from build123d import *

# Parameters (mm, degrees)
BOSS_EXTRUDE1_DEPTH = 33.65


with BuildPart() as part:
    # Sketch1 → Boss-Extrude1 (new body)
    with BuildSketch(Plane.XY):
        with BuildLine():
            Line((8.581782676, 84.338354997), (9.626750626, 92.275674602))
            ThreePointArc((9.626750626, 92.275674602), (8.629643832, 95.734969819), (5.415162452, 97.356097457))
            ThreePointArc((5.415162452, 97.356097457), (0, 97.506582836), (-5.415162452, 97.356097457))
            ThreePointArc((-5.415162452, 97.356097457), (-8.629643832, 95.734969819), (-9.626750626, 92.275674602))
            Line((-9.626750626, 92.275674602), (-8.581782676, 84.338354997))
            ThreePointArc((-8.581782676, 84.338354997), (-7.004465647, 81.471525738), (-3.902214001, 80.431009648))
            ThreePointArc((-3.902214001, 80.431009648), (0, 80.525614479), (3.902214001, 80.431009648))
            ThreePointArc((3.902214001, 80.431009648), (7.004465647, 81.471525738), (8.581782676, 84.338354997))
        make_face()
        with BuildLine():
            Line((-8.139583334, 92.47146389), (-7.094615384, 84.534144285))
            ThreePointArc((-7.094615384, 84.534144285), (-6.043070698, 82.622924779), (-3.974902934, 81.929247386))
            ThreePointArc((-3.974902934, 81.929247386), (0, 82.025614479), (3.974902934, 81.929247386))
            ThreePointArc((3.974902934, 81.929247386), (6.043070698, 82.622924779), (7.094615384, 84.534144285))
            Line((7.094615384, 84.534144285), (8.139583334, 92.47146389))
            ThreePointArc((8.139583334, 92.47146389), (7.474845471, 94.777660702), (5.331857885, 95.85841246))
            ThreePointArc((5.331857885, 95.85841246), (0, 96.006582836), (-5.331857885, 95.85841246))
            ThreePointArc((-5.331857885, 95.85841246), (-7.474845471, 94.777660702), (-8.139583334, 92.47146389))
        make_face(mode=Mode.SUBTRACT)
    extrude(amount=BOSS_EXTRUDE1_DEPTH)


solid = part.part
The listing builds one solid part. Answer for the finished solid, in the listing's coordinates (mm). A direction names the side the tool comes from. Coordinates: 2 decimals unless noted, no trailing zeros. Order: outer loops, then holes, each group sorted by start corner. A loop starts at its lowest first (then second) coordinate and runs counter-clockwise, first axis right, second up. Notation, with made-up numbers: M 76.25,42.25 L 82.25,42.25 A17 ccw 82.25,49.25 Z; hole C -11.5,73 d11. An arc over 180 degrees is marked long. Use CSV: the item, a comma, the result in double quotes.
Q1. Determine the mould class of faces 1 (the flat face through (0, 97, 0)), 2 (the cylindrical face through (-7.04, 81.5, 16.59)), 3 (the cylindrical face through (-0.056, 82.026, 16.589)) for opening direction Y: pulls with the +Y half, pulls with the -Y half, needs draft (parallel to the pull), parting line crosses it, or undercut.
Here are the results:
face 1,"needs draft"
face 2,"pulls with the -Y half"
face 3,"undercut"
Q2. Section A-A (x = 6.5) is taken. Determine the outline of the cut face in (y, z), then the cut area to 3 significant figures.
Here are the results:
outline,"M 81.11,0 L 83.1,0 L 83.1,33.65 L 81.11,33.65 Z; M 95.55,0 L 97.16,0 L 97.16,33.65 L 95.55,33.65 Z"
area,"121 mm2"
Q3. Straight lines are drawn through the part: L1, parallel to Y at x = 1, z = 20; L2, parallel to X at y = 86.25, z = 20; L3, parallel to X at y = 89, z = 11. For each, find the intervals that lie inside material, in ascending order.
Here are the results:
L1,"80.52 to 82.02, 96 to 97.5"
L2,"-8.83 to -7.32, 7.32 to 8.83"
L3,"-9.2 to -7.68, 7.68 to 9.2"
Q4. Given pin 1 Ø6 at (x, y) = (5.5, 82.5) entering from -Z; pin 2 Ø1 at (x, z) = (1.5, 22.5) entering from -Y; pin 3 Ø6 at (y, z) = (89, 20) entering from +X; pin 4 Ø8 at (x, z) = (-7, 4.5) entering from +Y, each flat-ended and moving along its own axis, determine where each tip first touches the part or whether it passes through.
Here are the results:
pin 1,"z = 0"
pin 2,"y = 80.5"
pin 3,"x = 9.59"
pin 4,"y = 97.46"
Q5. Section B-B (y = 93.75) is taken. Determine the outline of the cut face in (x, z).
Here are the results:
outline,"M -9.58,0 L -8.03,0 L -8.03,33.65 L -9.58,33.65 Z; M 8.03,0 L 9.58,0 L 9.58,33.65 L 8.03,33.65 Z"
Q6. A tool of negligible diameter and unlimited length cuts with its end or side. For faces 4 (the flat face through (-9.11, 88.36, 16.59)), 5 (the cylindrical face through (7.5, 94.75, 16.59)), from which of +Z, -Z, +X, -X, +Y, -Y can it reach the whole face along a straight path? Write none if from no direction.
Here are the results:
face 4,"+Z, -Z, -X, -Y"
face 5,"+Z, -Z"
Q7. Section C-C (z = 15) is taken. Determine the outline of the cut face in (x, y), then the cut area to 3 significant figures.
Here are the results:
outline,"M -9.63,92.28 L -8.58,84.34 A4.5 ccw -3.9,80.43 A80.53 cw 3.9,80.43 A4.5 ccw 8.58,84.34 L 9.63,92.28 A4.5 ccw 5.42,97.36 A97.51 ccw -5.42,97.36 A4.5 ccw Z; hole M -8.14,92.47 L -7.09,84.53 A3 ccw -3.97,81.93 A82.03 cw 3.97,81.93 A3 ccw 7.09,84.53 L 8.14,92.47 A3 ccw 5.33,95.86 A96.01 ccw -5.33,95.86 A3 ccw Z"
area,"87.2 mm2"
